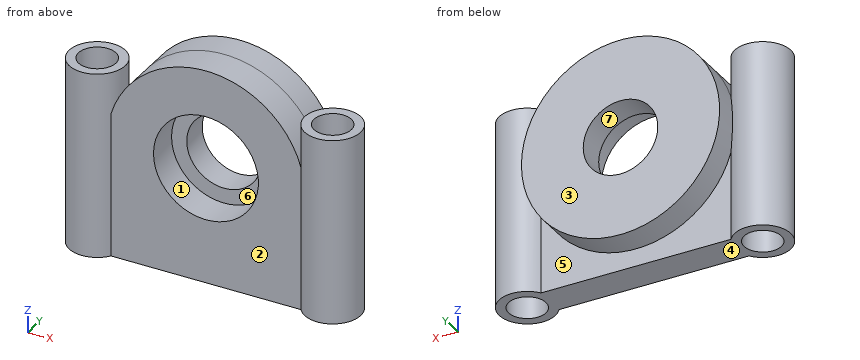
Autodesk Inventor part; units mm, degrees
ref_plane "YZ Plane" through (0, 0, 0) normal (1, 0, 0) x (0, 1, 0)
ref_plane "XZ Plane" through (0, 0, 0) normal (0, 1, 0) x (-1, 0, 0)
ref_plane "XY Plane" through (0, 0, 0) normal (0, 0, 1) x (1, 0, 0)
sketch "Sketch1" plane through (0, 0, 0) normal (0, 1, 0) x (-1, 0, 0)
  circle A0 centre (0, 0) radius 11.25
  arc A1 (21.25, 0) -> (-21.25, 0) centre (0, 0) ccw
  line L0 (0, -140) -> (21.25, -140)
  line L1 (21.25, -140) -> (-21.25, -140)
  line L2 (-21.25, -140) -> (-21.25, 0)
  line L3 (21.25, -140) -> (21.25, 0)
  dimension "d0" = 22.5
extrude "Extrusion1" add sketch "Sketch1" along normal blind 7
sketch "Sketch2" plane through (0, 7, 0) normal (0, 1, 0) x (1, 0, 0)
  circle A0 centre (0, 0) radius 11.25
  circle A1 centre (0, 0) radius 21.25
  circle A2 centre (0, 0) radius 8
  dimension "d5" = 16
extrude "Extrusion2" add sketch "Sketch2" along normal blind 6 contours A0 | A1
sketch "Sketch3" plane through (0, 7, 0) normal (0, 1, 0) x (1, 0, 0)
  point P0 (0, 0)
sketch "Sketch4" plane through (21.25, 0, -140) normal (0, 0, -1) x (-1, 0, 0)
  line L0 (0, 0) -> (42.5, 0)
  line L1 (42.5, 0) -> (42.5, 7)
  line L2 (0, 7) -> (42.5, 7)
  line L3 (0, 0) -> (0, 7)
  point P0 (21.25, 0)
extrude "Extrusion3" cut sketch "Sketch4" against normal blind 115
sketch "Sketch5" plane through (21.25, 0, -25) normal (0, 0, -1) x (-1, 0, 0)
  line L0 (0, 0) -> (0, 7)
  line L1 (0, 3.5) -> (-4, 3.5)
  circle A0 centre (-4, 3.5) radius 4
  circle A1 centre (-4, 3.5) radius 6
  line L2 (42.5, 0) -> (42.5, 7)
  line L3 (42.5, 3.5) -> (46.5, 3.5)
  circle A2 centre (46.5, 3.5) radius 4
  circle A3 centre (46.5, 3.5) radius 6
  point P0 (21.25, 0)
  dimension "d10" = 4
  dimension "d11" = 8
  dimension "d12" = 12
  dimension "d13" = 4
  dimension "d14" = 12
extrude "Extrusion4" add sketch "Sketch5" against normal blind 40
properties part number "wheel_stabilizer"
Build history of the part. All positions in model axes, mm. Face numbers are marked on the shaded views. A direction names the side the tool comes from. Give positions to 0.01 mm unless a question says otherwise; leave off trailing zeros. Loops run counter-clockwise (first coordinate to the right, second up) from the corner with the lowest first, then second, coordinate; pieces in that order, holes last.
Item 1: Flat gauge pins, fed straight in: pin 1 (3.5 mm diameter, centred on x = 23, y = 3, fed in from +Z); pin 2 (10 mm diameter, centred on x = 1, z = -3.5, fed in from -Y); pin 3 (1.5 mm diameter, centred on x = -20, y = 9, fed in from -Z); pin 4 (4 mm diameter, centred on y = 2.5, z = 8, fed in from +X). Where does each tip first touch, or does it go through?
Answers follow:
pin 1: stops at z = 15
pin 2: stops at y = 7
pin 3: stops at z = -9
pin 4: stops at x = 31.25
Item 2: Slice it at C-C, the plane z = 4.5. List the corners of the cut face in (x, y), and give its area (4 significant figures).
Answers follow:
outline: (-20.77, 7.49) arc R6 ccw (long way) to (-20.38, 0) - (-10.31, 0) - (-10.31, 7) - (-6.61, 7) - (-6.61, 13) - (-20.77, 13) - close; (6.61, 7) - (10.31, 7) - (10.31, 0) - (20.38, 0) arc R6 ccw (long way) to (20.77, 7.49) - (20.77, 13) - (6.61, 13) - close; hole circle Ø8 at (-25.25, 3.5); hole circle Ø8 at (25.25, 3.5)
area: 425.5 mm2
Item 3: Pull direction Z, two halves, no side cores. Call the marked faces 4, 5, 6 and 7: released by +Z, released by -Z, zero draft, split by the parting line, or undercut.
Answers follow:
face 4: released by -Z
face 5: zero draft
face 6: undercut
face 7: undercut
Item 4: Slice it at D-D, the plane z = -17. List the corners of the cut face in (x, y), and give its area (3 significant figures).
Answers follow:
outline: (-20.38, 0) - (20.38, 0) arc R6 ccw (long way) to (20.38, 7) - (12.75, 7) - (12.75, 13) - (-12.75, 13) - (-12.75, 7) - (-20.38, 7) arc R6 ccw (long way) to start; hole circle Ø8 at (-25.25, 3.5); hole circle Ø8 at (25.25, 3.5)
area: 553 mm2
Item 5: Drill centre lines: line 1 (X direction, y = 4.75, z = -12.5); line 2 (Y direction, x = 25, z = -9); line 3 (Z direction, x = 0, y = 10.6). Where is each one in solid material? Low to high.
Answers follow:
line 1: x = -31.12 to -29.05, -21.45 to 21.45, 29.05 to 31.12
line 2: y = -2.49 to -0.49, 7.49 to 9.49
line 3: z = -21.25 to -8, 8 to 21.25
Item 6: Slice it at B-B, the plane x = -25.25. List the corners of the cut face in (y, z), and give its area (3 significant figures).
Answers follow:
outline: (-2.5, -25) - (-0.5, -25) - (-0.5, 15) - (-2.5, 15) - close; (7.5, -25) - (9.5, -25) - (9.5, 15) - (7.5, 15) - close
area: 160 mm2
Item 7: Slice it at A-A, the plane y = 3.5. List the corners of the cut face in (x, z), and give its area (3 significant figures).
Answers follow:
outline: (-31.25, -25) - (-29.25, -25) - (-29.25, 15) - (-31.25, 15) - close; (-21.25, -25) - (21.25, -25) - (21.25, 15) - (19.25, 15) - (19.25, 9) arc R21.25 ccw to (-19.25, 9) - (-19.25, 15) - (-21.25, 15) - close; (29.25, -25) - (31.25, -25) - (31.25, 15) - (29.25, 15) - close; hole circle Ø22.5 at (0, 0)
area: 1,570 mm2
Item 8: Which spindle directions (+Z, -Z, +X, -X, +Y, -Y) get a long thin tool onto all of the face, cutting with end or side? Do the marked faces 1, 2 and 3. Say none if no direction does.
Answers follow:
face 1: -Y
face 2: +Z, -Z, -Y
face 3: +Z, -Z, +X, -X, +Y
